Design review of the part built by this model. Coordinates are the model's own, in mm. Coordinates: 2 decimals unless noted, no trailing zeros. Order: outer loops, then holes, each group sorted by start corner. A loop starts at its lowest first (then second) coordinate and runs counter-clockwise, first axis right, second up. Notation, with made-up numbers: M 75,-4.5 L 124,-4.5 A27 cw 124,13.5 Z; hole C -1.75,19.5 d7. An arc over 180 degrees is marked long. Answer in a Markdown table with one row per item.
from build123d import *

# Parameters (mm, degrees)
F3_R    = 2.54
F4_SIZE = 2.54


with BuildPart() as f2:
    # F0 (on Front) → F2 (revolve)
    with BuildSketch(Plane.XZ):
        Polygon((2.032, 12.7), (2.032, 0), (19.05, 0), (11.43, 25.4), (5.08, 25.4), (5.08, 17.054286), align=None)
    revolve(axis=Axis((0, 0, 16.681224), (0, 0, 1)))

    # F3
    f3_edges = [f2.edges().sort_by_distance(p)[0] for p in [
        (-11.43, 0, 25.4),
        (-5.08, 0, 25.4),
        (-19.05, 0, 0),
    ]]
    fillet(f3_edges, radius=F3_R)

    # F4
    f4_edges = [f2.edges().sort_by_distance(p)[0] for p in [
        (-2.032, 0, 0),
    ]]
    chamfer(f4_edges, length=F4_SIZE)


solid = f2.part
(1) Add section A-A, the plane x = 0. Give the boundary of the cut face in (y, z).
Return value:
| item | result |
|---|---|
| outline | M -18.07,3.27 A2.54 ccw -15.64,0 L -4.57,0 L -2.03,2.54 L -2.03,12.7 L -5.08,17.05 L -5.08,22.86 A2.54 ccw -7.62,25.4 L -9.54,25.4 A2.54 ccw -11.97,23.59 Z; M 2.03,2.54 L 4.57,0 L 15.64,0 A2.54 ccw 18.07,3.27 L 11.97,23.59 A2.54 ccw 9.54,25.4 L 7.62,25.4 A2.54 ccw 5.08,22.86 L 5.08,17.05 L 2.03,12.7 Z |
(2) Draft analysis for pull direction X (two halves, no side actions). For faces 1 (the conical face through (-0.55, -2.46, 13.4)), 2 (the cylindrical face through (-0.661, 5.037, 19.917)), 3 (the conical face through (-1.8, 13.5, 18.1)), 4 (the flat face through (-3, 4, 0)), state which applies: pulls with the +X half, pulls with the -X half, needs draft (parallel to the pull), parting line crosses it, or undercut.
Return value:
| item | result |
|---|---|
| face 1 | undercut |
| face 2 | undercut |
| face 3 | parting line crosses it |
| face 4 | needs draft |
(3) For line 1 along Y through (x, z) = (0, 8.5); line 2 along Y through (x, z) = (0, 9); line 3 along X through (y, z) = (-11, 6.25), list the stretches that pass through material, from the lowest coordinate up. Write a range as from..to.
Return value:
| item | result |
|---|---|
| line 1 | y = -16.5..-2.03, 2.03..16.5 |
| line 2 | y = -16.35..-2.03, 2.03..16.35 |
| line 3 | x = -13.19..13.19 |
(4) Insertion check: pin 1 Ø8 at (x, z) = (-6.5, 9) entering from -Y; pin 2 Ø1 at (x, z) = (5, 11) entering from +Y; pin 3 Ø6 at (x, z) = (4.5, 18) entering from +Y. Each pin has a flat end and moves straight along its axis. Give the tip position at first contact, or say it passes through.
Return value:
| item | result |
|---|---|
| pin 1 | stops at y = -16.82 |
| pin 2 | stops at y = 15.16 |
| pin 3 | stops at y = 14.12 |
(5) Add section D-D, the plane z = 14. Give the boundary of the cut face in (x, y).
Return value:
| item | result |
|---|---|
| outline | C 0,0 d29.7; hole C 0,0 d5.88 |
(6) Add section C-C, the plane z = 7. Give the boundary of the cut face in (x, y), and give its area (3 significant figures).
Return value:
| item | result |
|---|---|
| outline | C 0,0 d33.9; hole C 0,0 d4.06 |
| area | 890 mm2 |
